```python
from build123d import *

# Parameters (mm, degrees)
F0_R      = 9.525
F1_DEPTH  = 50.8
F3_D      = 10.4902
F3_DEPTH  = 41.275
F3_TIP    = 3.1515740329
F5_D      = 3.4544
F7_DEPTH  = 0.79375
F8_SIZE   = 0.79375
F10_DEPTH = 25.4


with BuildPart() as f1:
    # F0 (on Top) → F1 (new body)
    with BuildSketch(Plane.XY):
        Circle(F0_R)
    extrude(amount=F1_DEPTH)

    # F3
    with Locations(Plane.XY.offset(50.8)):
        with Locations((0, 0)):
            Hole(F3_D / 2, depth=F3_DEPTH)
            with Locations((0, 0, -(F3_DEPTH + F3_TIP / 2))):  # 118° drill point
                Cone(0, F3_D / 2, F3_TIP, mode=Mode.SUBTRACT)

    # F5 (through all)
    with Locations(Plane(origin=(0, 0, 0), x_dir=(1, 0, 0), z_dir=(0, 0, -1))):
        with Locations((0, 0)):
            Hole(F5_D / 2)

    # F6 (on face) → F7 (cut)
    with BuildSketch(Plane.XY.offset(50.8)):
        with BuildLine():
            ThreePointArc((-4.7278053569, -2.2713279193), (-4.5423898454, 2.62255), (-0.396875, 5.2300635029))
            Line((-0.396875, 5.2300635029), (-0.396875, 9.5167281791))
            ThreePointArc((-0.396875, 9.5167281791), (-8.248891971, 4.7625), (-8.440165864, -4.4146602574))
            Line((-8.440165864, -4.4146602574), (-4.7278053569, -2.2713279193))
        make_face()
        with BuildLine():
            Line((8.043290864, -5.1020679217), (4.3309303569, -2.9587355836))
            ThreePointArc((4.3309303569, -2.9587355836), (0, -5.2451), (-4.3309303569, -2.9587355836))
            Line((-4.3309303569, -2.9587355836), (-8.043290864, -5.1020679217))
            ThreePointArc((-8.043290864, -5.1020679217), (0, -9.525), (8.043290864, -5.1020679217))
        make_face()
        with BuildLine():
            ThreePointArc((0.396875, 5.2300635029), (3.8466038965, 3.5657695486), (5.2451, 0))
            ThreePointArc((5.2451, 0), (5.1141414669, -1.1647450649), (4.7278053569, -2.2713279193))
            Line((4.7278053569, -2.2713279193), (8.440165864, -4.4146602574))
            ThreePointArc((8.440165864, -4.4146602574), (9.2498163456, -2.2729985862), (9.525, 0))
            ThreePointArc((9.525, 0), (6.8740766425, 6.5933826912), (0.396875, 9.5167281791))
            Line((0.396875, 9.5167281791), (0.396875, 5.2300635029))
        make_face()
    extrude(amount=-F7_DEPTH, mode=Mode.SUBTRACT)

    # F8
    f8_edges = [f1.edges().sort_by_distance(p)[0] for p in [
        (8.248892, -4.7625, 50.8),
        (0, 9.525, 50.8),
        (-8.248892, -4.7625, 50.8),
        (4.54239, -2.62255, 50.8),
        (-4.54239, -2.62255, 50.8),
        (0, 5.2451, 50.8),
    ]]
    chamfer(f8_edges, length=F8_SIZE)

    # F9 (on Front) → F10 (cut)
    with BuildSketch(Plane.XZ):
        with BuildLine():
            ThreePointArc((3.175, 52.54625), (0, 55.72125), (-3.175, 52.54625))
            Line((-3.175, 52.54625), (-3.175, 9.525))
            ThreePointArc((-3.175, 9.525), (0, 6.35), (3.175, 9.525))
            Line((3.175, 9.525), (3.175, 52.54625))
        make_face()
    extrude(amount=F10_DEPTH, mode=Mode.SUBTRACT)


solid = f1.part
```
The model under review builds one solid part; all positions refer to its coordinate system, in mm. A direction names the side the tool comes from. Round coordinates to 2 decimals unless told otherwise and drop trailing zeros. Loops run counter-clockwise (first coordinate to the right, second up) from the corner with the lowest first, then second, coordinate; pieces in that order, holes last.
1) Tool access review of faces 1 (the face through (-2.16, 0, 7.42)), 2 (the face through (-6.61, -3.36, 50.41)), 3 (the face through (-0.183, 5.242, 29.482)): name each direction out of +Z, -Z, +X, -X, +Y, -Y from which nothing blocks a thin tool from reaching the whole face with its end or side.
Values follow:
face 1: +Z, -Y
face 2: +Z, -X, +Y
face 3: +Z
2) Consider section A-A on y = 8. State the section outline as (x, z) points.
Values follow:
outline: (-5.17, 0) - (5.17, 0) - (5.17, 50.01) - (0.4, 50.01) - (0.4, 50.8) - (-0.4, 50.8) - (-0.4, 50.01) - (-5.17, 50.01) - close
3) The part is to be moulded in two halves that separate along X. For faces 4 (the face through (6.56, -3.33, 50.41)), 5 (the face through (2.2, 0, 7.5)), 6 (the face through (-6.4, -3.7, 50.8)), 7 (the face through (-7.9, -4.56, 50.41)), say which applies: pulls with the +X half, pulls with the -X half, needs draft (parallel to the pull), parting line crosses it, or undercut.
Values follow:
face 4: pulls with the +X half
face 5: undercut
face 6: needs draft
face 7: pulls with the -X half
4) Wall thickness on line 1 along Y through (x, z) = (0, 4) (3 decimals); line 2 along X through (y, z) = (0, 29.5) (3 decimals); line 3 along Y through (x, z) = (0, 23) (3 decimals): over which ranges is each line inside the solid? List them lowest first.
Values follow:
line 1: y = -9.525 to -1.727, 1.727 to 9.525
line 2: x = -9.525 to -5.245, 5.245 to 9.525
line 3: y = 5.245 to 9.525
5) Clearance check with flat-ended pins moving along their axes: P1, Ø1, axis at x = -2.5, y = 1.5, coming from the +Z side; P2, Ø4.5, axis at x = -7, y = 3, coming from the +Z side; P3, Ø0.6, axis at y = 8, z = 50.5, coming from the -X side. State where each tip first meets the part, or that it passes through.
Values follow:
P1: stops at z = 8.43
P2: stops at z = 50.01
P3: stops at x = -0.4
6) Consider section C-C on x = -6.5. State the section outline as (y, z) points, then the cut area to 3 significant figures.
Values follow:
outline: (-6.96, 0) - (6.96, 0) - (6.96, 50.01) - (-3.29, 50.01) - (-3.29, 50.8) - (-4.21, 50.8) - (-4.21, 50.01) - (-6.96, 50.01) - close
area: 697 mm2
7) Consider section B-B on z = 29. State the section outline as (x, y) points (3 decimals).
Values follow:
outline: (-3.175, -8.98) - (-3.175, -4.175) arc R5.245 cw (long way) to (3.175, -4.175) - (3.175, -8.98) arc R9.525 ccw (long way) to start
